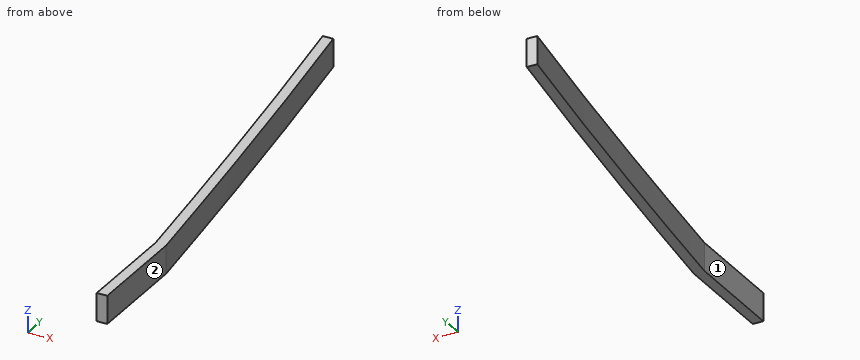
```python
from build123d import *

# Parameters (mm, degrees)
BOSS_EXTRUDE1_DEPTH      = 6.35
BOSS_EXTRUDE1_DEPTH_BACK = 6.35


with BuildPart() as part:
    # Sketch3 → Boss-Extrude1 (new, two sides: drawn at the far end of the back side and taken through both)
    with BuildSketch(Plane.XY.offset(-BOSS_EXTRUDE1_DEPTH_BACK)):
        with BuildLine():
            Line((25.930295497, 228.6), (30.692795497, 228.6))
            add(Edge.make_bspline(
                [(30.692795497, 228.6), (32.656671965, 216.59798975), (34.557493546, 204.585654572), (41.339553497, 160.498217254), (45.907919412, 128.375397263), (52.344898005, 80.136373161), (54.419889898, 64.046285851), (56.441032457, 47.840855492), (56.454490883, 47.732922744), (56.467945104, 47.625)],
                knots=[0.158181503, 0.158181503, 0.158181503, 0.158181503, 0.194666408, 0.194666408, 0.291999611, 0.291999611, 0.340666213, 0.340666213, 0.340992559, 0.340992559, 0.340992559, 0.340992559], degree=3))
            Line((56.467945104, 47.625), (56.467945104, 0))
            Line((56.467945104, 0), (51.705445104, 0))
            Line((51.705445104, 0), (51.705445104, 47.625))
            add(Edge.make_bspline(
                [(25.930295497, 228.6), (28.835110587, 210.988612906), (34.358497112, 175.720617461), (40.71056634, 131.542229957), (45.5050338, 96.160367974), (48.389330035, 74.025463782), (50.34888675, 58.533876957), (51.261329801, 51.213221833), (51.621113082, 48.307200473), (51.705445104, 47.625)],
                knots=[0.158553364, 0.158553364, 0.158553364, 0.158553364, 0.216147542, 0.273741721, 0.30253881, 0.3313359, 0.345734444, 0.352933717, 0.355143131, 0.355143131, 0.355143131, 0.355143131], degree=3))
        make_face()
    extrude(amount=BOSS_EXTRUDE1_DEPTH + BOSS_EXTRUDE1_DEPTH_BACK)


solid = part.part
```
The listing builds one solid part. Answer for the finished solid, in the listing's coordinates (mm). Face numbers are marked on the shaded views. A direction names the side the tool comes from. Coordinates: 2 decimals unless noted, no trailing zeros. Loops run counter-clockwise (first coordinate to the right, second up) from the corner with the lowest first, then second, coordinate; pieces in that order, holes last. Notation, with made-up numbers: M 83.5,80 L 96.5,80 A19 ccw 96.5,85 Z; hole C 3.25,40 d7. An arc over 180 degrees is marked long. Answer as a JSON object with one key per item and string values. Group by question number.
Item 1: Which of the six approach directions +Z, -Z, +X, -X, +Y, -Y give full straight-line access (tool end or side, diameter ignored) to the marked faces 1 and 2?
Item 2: Each of these flat-tipped pins is pushed along its axis until it touches: P1, Ø3, axis at y = 60.5, z = -4.5, coming from the +X side; P2, Ø4, axis at y = 90.5, z = -2.5, coming from the +X side. Where does it stop, or does it pass through?
Item 3: Consider L1, parallel to X at y = 31, z = 3; L2, parallel to X at y = 76, z = 3.25. Determine where each line is inside the solid, lowest interval first.
Item 4: Section A-A (y = 37.5) is taken. Write down the section's boundary in (x, z), and give its area (3 significant figures).
Solved:
{
 "1": {"face 1": "+Z, -Z, -X, -Y", "face 2": "+Z, -Z, +X, +Y, -Y"},
 "2": {"P1": "stops at x = 55.04", "P2": "stops at x = 51.22"},
 "3": {"L1": "x = 51.71 to 56.47", "L2": "x = 48.12 to 52.86"},
 "4": {"outline": "M 51.71,-6.35 L 56.47,-6.35 L 56.47,6.35 L 51.71,6.35 Z", "area": "60.5 mm2"}
}
